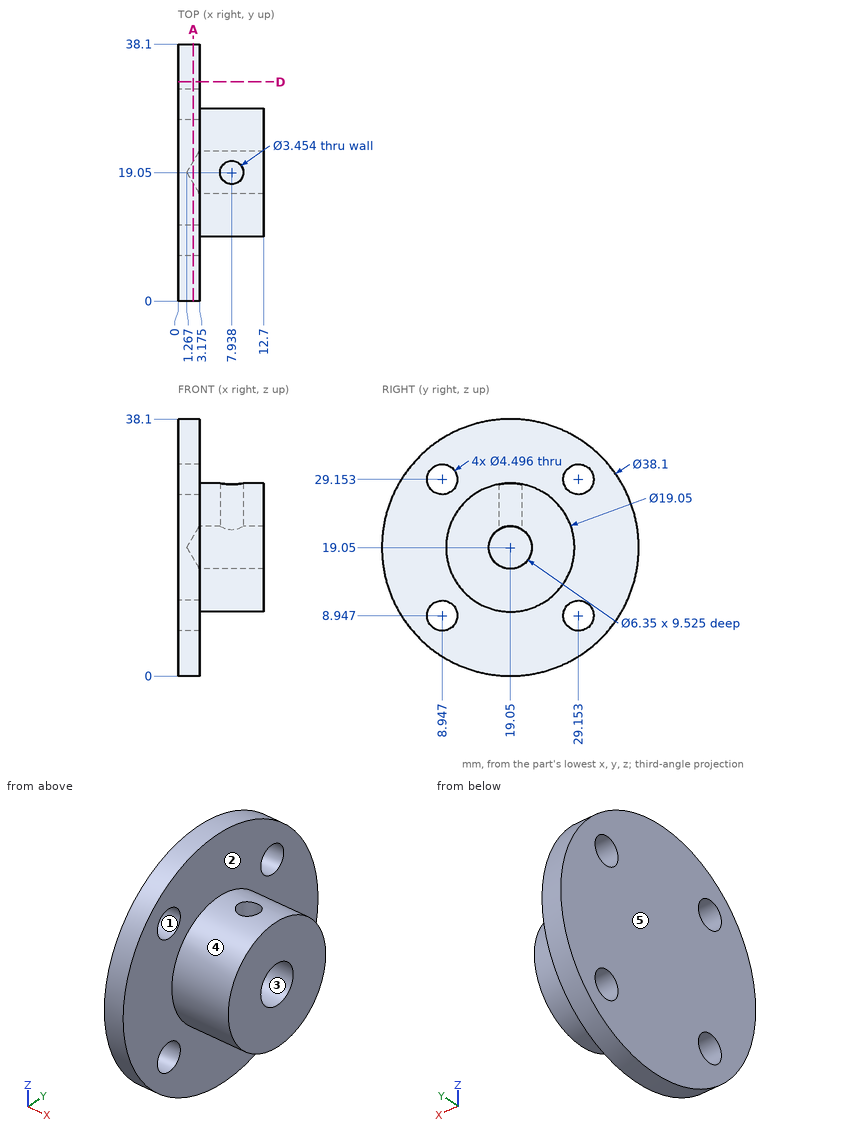
Input: dimensioned drawing with shaded views. Units: mm. Origin: part minimum x, y, z. A direction names the side the tool comes from. Give positions to 0.01 mm unless a question says otherwise; leave off trailing zeros. Loops run counter-clockwise (first coordinate to the right, second up) from the corner with the lowest first, then second, coordinate; pieces in that order, holes last. Notation, with made-up numbers: M 20,18.5 L 61,18.5 A30 cw 61,56.5 Z; hole C -3,-25.5 d5. An arc over 180 degrees is marked long. Put each result on its own line as item: value. Start each with the question number.
1) Pull-direction query (Z, two-part tool) for the marked faces 3, 4 and 5; classes: pulls with the +Z half, pulls with the -Z half, needs draft (parallel to the pull), parting line crosses it, or undercut.
2) Contact query for flat-ended pins moving along their axis: pin 1 (6 mm diameter, centred on x = 5.5, z = 10.5, fed in from +Y); pin 2 (7 mm diameter, centred on y = 29.15, z = 8.95, fed in from +X) (1 decimal); pin 3 (4.5 mm diameter, centred on x = 7.94, y = 19.05, fed in from -Z) (1 decimal). Output: stop coordinate, or through.
3) Access query for the marked faces 1 and 2. Directions: +Z, -Z, +X, -X, +Y, -Y. A direction counts if a zero-diameter tool reaches every point of the face in a straight line with its end or side. Return the directions, or none.
4) Cut plane D-D (y = 32.5). Output: boundary loops of the cut face in (x, z) (1 decimal).
5) Ray query, line 1 along Z through (x, y) = (1.75, 30) (1 decimal); line 2 along X through (y, z) = (31.5, 11.5) (1 decimal); line 3 along Z through (x, y) = (5.25, 19.05) (1 decimal). Return the intervals inside material, ascending.
6) Cut plane A-A (x = 2.25). Give the number of separate pieces and of enclosed holes in the cut face, then the cut area to 3 significant figures.
Verdict:
1. face 3: undercut
1. face 4: parting line crosses it
1. face 5: needs draft
2. pin 1: y = 36.9
2. pin 2: x = 3.2
2. pin 3: z = 9.5
3. face 1: +X, -X
3. face 2: +X
4. outline: M 0,5.6 L 3.2,5.6 L 3.2,32.5 L 0,32.5 Z
5. line 1: 3.5 to 6.9, 11 to 27.1, 31.2 to 34.6
5. line 2: 0 to 3.2
5. line 3: 9.5 to 15.9, 22.2 to 28.6
6. separate pieces: 1
6. enclosed holes: 5
6. area: 1,070 mm2
